```python
from build123d import *

# Parameters (mm, degrees)
F0_W = 40
F0_H = 40


with BuildPart() as f2:
    # F0 (on Top) → F2 section 0
    with BuildSketch(Plane.XY, mode=Mode.PRIVATE) as f2_s0:
        Rectangle(F0_W, F0_H)
    loft([f2_s0.sketch, Vertex(0, 0, 28.284271)])

    # F3: F2 across plane


with BuildPart() as f2_1:
    add(f2.part)
    add(f2.part.mirror(Plane.XY))


solid = f2_1.part
```
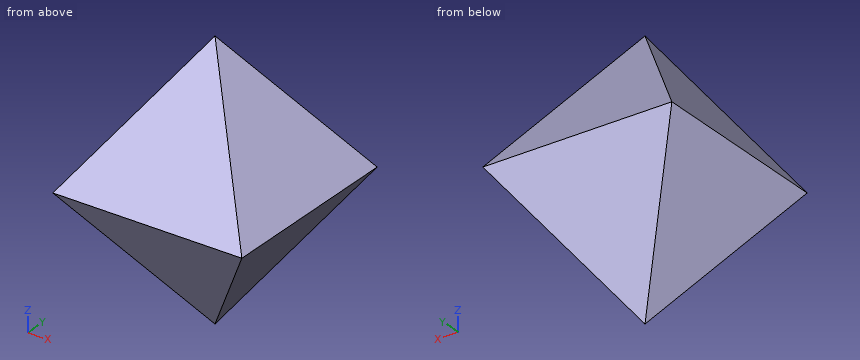
Part model, mm, in its own coordinate system. Round coordinates to 2 decimals unless told otherwise and drop trailing zeros. Write each loop counter-clockwise with the first axis right and the second up, starting at its lowest first coordinate (ties: lowest second). Pieces come first, ordered by that corner, then holes. Notation, with made-up numbers: M 28,-28 L 71,-28 A25 ccw 71,-11 Z; hole C 11,30 d8. An arc over 180 degrees is marked long. One line per question, with ' | ' between items.
(1) Probe line 1 along Y through (x, z) = (7, 18); line 2 along X through (y, z) = (-7, 10); line 3 along Z through (x, y) = (-8, 0). List the from-to ranges inside material, lowest first.
Answer key:
line 1: y = -7.27 to 7.27 | line 2: x = -12.93 to 12.93 | line 3: z = -16.97 to 16.97
(2) Saw through at C-C on z = 22.5. Write the cut outline in (x, y).
Answer key:
outline: M -4.09,-4.09 L 4.09,-4.09 L 4.09,4.09 L -4.09,4.09 Z
(3) Saw through at B-B on x = -10. Write the cut outline in (y, z), then the cut area to 3 significant figures.
Answer key:
outline: M -20,0 L -10,-14.14 L 10,-14.14 L 20,0 L 10,14.14 L -10,14.14 Z | area: 849 mm^2
(4) Saw through at D-D on z = -21. Write the cut outline in (x, y).
Answer key:
outline: M -5.15,-5.15 L 5.15,-5.15 L 5.15,5.15 L -5.15,5.15 Z
(5) Saw through at A-A on y = -5.5. Write the cut outline in (x, z), then the cut area to 3 significant figures.
Answer key:
outline: M -20,0 L -5.5,-20.51 L 5.5,-20.51 L 20,0 L 5.5,20.51 L -5.5,20.51 Z | area: 1,050 mm^2
(6) Pin check, flat tips, straight feed: pin 1 (1 mm diameter, centred on x = -12.5, y = 9.5, fed in from +Z); pin 2 (6 mm diameter, centred on x = -0.5, z = 15.5, fed in from -Y); pin 3 (2 mm diameter, centred on x = -5.5, y = 6, fed in from -Z). Stop position of each tip, or through.
Answer key:
pin 1: stops at z = 11.31 | pin 2: stops at y = -11.16 | pin 3: stops at z = -21.09
